The drawing under review shows one solid part. Ordinate dimensions are in mm from its lowest x, y, z. A direction names the side the tool comes from. Give positions to 0.01 mm unless a question says otherwise; leave off trailing zeros. Loops run counter-clockwise (first coordinate to the right, second up) from the corner with the lowest first, then second, coordinate; pieces in that order, holes last.
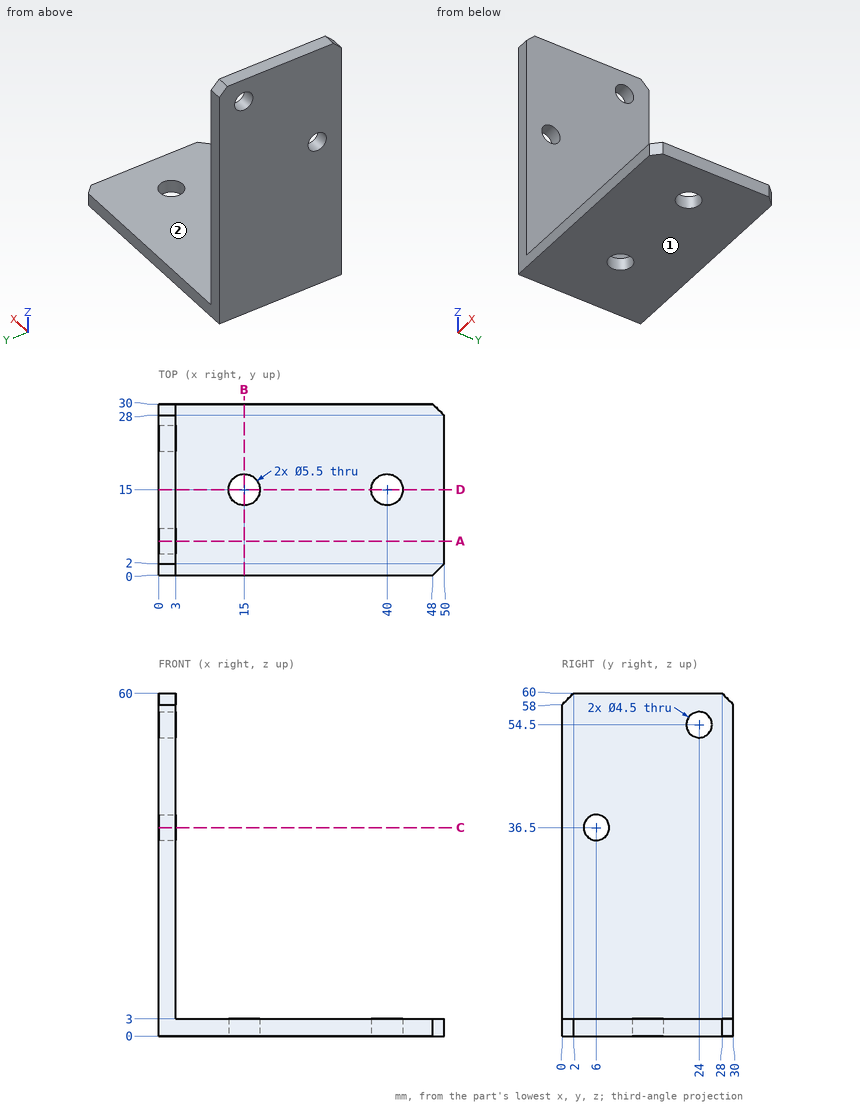
Item 1: Take a section at A-A on y = 6. Give the boundary of the cut face in (x, z).
Answer:
outline: (0, 0) - (50, 0) - (50, 3) - (3, 3) - (3, 34.25) - (0, 34.25) - close; (0, 38.75) - (3, 38.75) - (3, 60) - (0, 60) - close
Item 2: Take a section at D-D on y = 15. Give the boundary of the cut face in (x, z), and give its area (3 significant figures).
Answer:
outline: (0, 0) - (12.25, 0) - (12.25, 3) - (3, 3) - (3, 60) - (0, 60) - close; (17.75, 0) - (37.25, 0) - (37.25, 3) - (17.75, 3) - close; (42.75, 0) - (50, 0) - (50, 3) - (42.75, 3) - close
area: 288 mm2
Item 3: Take a section at B-B on x = 15. Give the boundary of the cut face in (y, z).
Answer:
outline: (0, 0) - (12.25, 0) - (12.25, 3) - (0, 3) - close; (17.75, 0) - (30, 0) - (30, 3) - (17.75, 3) - close
Item 4: Tool access review of the marked faces 1 and 2: name each direction out of +Z, -Z, +X, -X, +Y, -Y from which nothing blocks a thin tool from reaching the whole face with its end or side.
Answer:
face 1: -Z, +X, -X, +Y, -Y
face 2: +Z, +X, +Y, -Y
Item 5: Clearance check with flat-ended pins moving along their axes: pin 1 Ø7 at (y, z) = (6, 36.5) entering from -X; pin 2 Ø6.5 at (x, y) = (15, 15) entering from +Z; pin 3 Ø12 at (y, z) = (13.5, 39.5) entering from +X. State where each tip first meets the part, or that it passes through.
Answer:
pin 1: stops at x = 0
pin 2: stops at z = 3
pin 3: stops at x = 3
Item 6: Take a section at C-C on z = 36.5. Give the boundary of the cut face in (x, y), and give its area (3 significant figures).
Answer:
outline: (0, 0) - (3, 0) - (3, 3.75) - (0, 3.75) - close; (0, 8.25) - (3, 8.25) - (3, 30) - (0, 30) - close
area: 76.5 mm2
Item 7: For L1, parallel to Z at x = 0.6, y = 6; L2, parallel to Y at x = 40, z = 2.15; L3, parallel to X at y = 21, z = 16, list the stretches that pass through material, from the lowest coordinate up.
Answer:
L1: z = 0 to 34.25, 38.75 to 60
L2: y = 0 to 12.25, 17.75 to 30
L3: x = 0 to 3
